```python
from build123d import *

# Parameters (mm, degrees)
F0_W     = 360
F0_H     = 360
F1_DEPTH = 2
F0_W_2   = 366
F0_H_2   = 366
F2_DEPTH = 5
F3_W     = 34
F3_H     = 3
F4_DEPTH = 25


with BuildPart() as f1:
    # F0 (on Top) → F1 (new body)
    with BuildSketch(Plane.XY):
        Rectangle(F0_W, F0_H)
    extrude(amount=F1_DEPTH)

    # F0 (on Top) → F2 (join)
    with BuildSketch(Plane.XY):
        Rectangle(F0_W_2, F0_H_2)
        Rectangle(F0_W, F0_H, mode=Mode.SUBTRACT)
    extrude(amount=F2_DEPTH)

    # F3 (on face) → F4 (intersect)
    with BuildSketch(Plane.XY.offset(5)):
        Polygon((17, -92.5), (17, -17), (-17, -17), (-17, -92.5), (-32, -87.5), (-32, -112.5), (-17, -107.5), (-17, -180), (17, -180), (17, -107.5), (32, -112.5), (32, -87.5), align=None)
        with Locations((0, -181.5)):
            Rectangle(F3_W, F3_H)
    extrude(amount=-F4_DEPTH, mode=Mode.INTERSECT)


solid = f1.part
```
The listing builds one solid part. Answer for the finished solid, in the listing's coordinates (mm). A direction names the side the tool comes from. Give positions to 0.01 mm unless a question says otherwise; leave off trailing zeros. Write each loop counter-clockwise with the first axis right and the second up, starting at its lowest first coordinate (ties: lowest second). Pieces come first, ordered by that corner, then holes. Notation, with made-up numbers: (43, -14.75) - (70, -14.75) arc R33 ccw to (70, 16.25) - close; hole circle Ø7 at (15.5, -25.75). An arc over 180 degrees is marked (long way). Use one line per item in the form item = value. Start each with the question number.
1) Find section B-B on z = 0.85. Determine the outline of the cut face in (x, y).
2) Consider line 1 along Y through (x, z) = (-1, 3); line 2 along Z through (x, y) = (-2, -79); line 3 along X through (y, z) = (-139, 0.35). Determine where each line is inside the solid, lowest interval first. Write a range as from..to.
3) Find section A-A on y = -109.5. Determine the outline of the cut face in (x, z).
4) Find section C-C on x = 13.5. Determine the outline of the cut face in (y, z), plus the area to 3 significant figures.
5) The mould has two halves that part along X. Classify faces 1 (the face through (24.395, -109.965, 1.014)), 2 (the face through (-24.395, -90.035, 1.014)), 3 (the face through (0, -181, 5)): pulls with the +X half, pulls with the -X half, needs draft (parallel to the pull), parting line crosses it, or undercut.
6) A tool of negligible diameter and unlimited length cuts with its end or side. For faces 4 (the face through (0, -97, 2)), 5 (the face through (-24.605, -110.035, 1.014)), 6 (the face through (24.605, -89.965, 1.014)), from which of +Z, -Z, +X, -X, +Y, -Y can it reach the whole face along a straight path? Write none if from no direction.
7) Flat-ended cylindrical pins translate along their axes: pin 1 Ø1.5 at (x, z) = (4, 4) entering from +Y; pin 2 Ø1.6 at (y, z) = (-56, 1) entering from -X; pin 3 Ø2 at (y, z) = (-51, 1.5) entering from +X. Find the tip coordinate at first contact, or state that the pin passes through.
8) Find section D-D on y = -37. Determine the outline of the cut face in (x, z), plus the area to 3 significant figures.
Geometry results:
q1.outline = (-32, -112.5) - (-17, -107.5) - (-17, -183) - (17, -183) - (17, -107.5) - (32, -112.5) - (32, -87.5) - (17, -92.5) - (17, -17) - (-17, -17) - (-17, -92.5) - (-32, -87.5) - close
q2.line_1 = -183..-180
q2.line_2 = 0..2
q2.line_3 = -17..17
q3.outline = (-32, 0) - (-23, 0) - (-23, 2) - (-32, 2) - close; (-17, 0) - (17, 0) - (17, 2) - (-17, 2) - close; (23, 0) - (32, 0) - (32, 2) - (23, 2) - close
q4.outline = (-183, 0) - (-17, 0) - (-17, 2) - (-180, 2) - (-180, 5) - (-183, 5) - close
q4.area = 341 mm2
q5.face_1 = undercut
q5.face_2 = undercut
q5.face_3 = needs draft
q6.face_4 = +Z, +X, -X, +Y
q6.face_5 = +Z, -Z, -Y
q6.face_6 = +Z, -Z, +Y
q7.pin_1 = -180
q7.pin_2 = -17
q7.pin_3 = 17
q8.outline = (-17, 0) - (17, 0) - (17, 2) - (-17, 2) - close
q8.area = 68.0 mm2
